```python
from build123d import *

# Parameters (mm, degrees)
SKETCH_1_W      = 134.3
SKETCH_1_H      = 22
EXTRUDE_1_DEPTH = 8
SKETCH_2_W      = 4
SKETCH_2_H      = 8
EXTRUDE_2_DEPTH = 130


with BuildPart() as part:
    # 草图1 → 凸台-拉伸1 (new body)
    with BuildSketch(Plane(origin=(0, 0, 0), x_dir=(1, 0, 0), z_dir=(0, 1, 0))):
        Rectangle(SKETCH_1_W, SKETCH_1_H)
    extrude(amount=EXTRUDE_1_DEPTH)

    # 草图2 → 凸台-拉伸2 (add)
    with BuildSketch(Plane.XY):
        with Locations((-17, 4)):
            Rectangle(SKETCH_2_W, SKETCH_2_H)
    extrude(amount=EXTRUDE_2_DEPTH)


solid = part.part
```
Design review of the part built by this model. Coordinates are the model's own, in mm. A direction names the side the tool comes from. Coordinates: 2 decimals unless noted, no trailing zeros. Write each loop counter-clockwise with the first axis right and the second up, starting at its lowest first coordinate (ties: lowest second). Pieces come first, ordered by that corner, then holes.
1) Add section B-B (x = -40). Write out the cut boundary in (y, z).
2) To check wall thickness, follow L1, parallel to X at y = 4.75, z = 101; L2, parallel to Z at x = 26.5, y = 7.75. State the ranges of each line that lie inside material, in increasing order.
3) Add section C-C (z = 82). Write out the cut boundary in (x, y), plus the area to 3 significant figures.
4) Machinability: for faces 1 (the flat face through (25, 4, 11)), 2 (the flat face through (67.15, 4, 0)), 3 (the flat face through (-19, 4, 70)), which of the approach directions +Z, -Z, +X, -X, +Y, -Y give a long, thin tool a straight path to every point of the face, cutting with its end or side? Answer none if there is none.
5) Insertion check: pin 1 (4 mm diameter, centred on y = 4.5, z = 96, fed in from -X); pin 2 (3 mm diameter, centred on x = -37.5, y = 3.5, fed in from +Z). Each pin has a flat end and moves straight along its axis. Give the tip position at first contact, or say it passes through.
6) Mouldability with a two-part tool opening along Y and no side actions: class faces 4 (the flat face through (-5, 0, 7)), 5 (the flat face through (-5, 8, 7)), 6 (the flat face through (-1, 4, -11)) as +Y half, -Y half, draft (parallel to the pull), parting line (faces both ways), or undercut.
7) Add section A-A (y = 6.75). Write out the cut boundary in (x, z), plus the area to 3 significant figures.
Check result:
1. outline: (0, -11) - (8, -11) - (8, 11) - (0, 11) - close
2. L1: x = -19 to -15
2. L2: z = -11 to 11
3. outline: (-19, 0) - (-15, 0) - (-15, 8) - (-19, 8) - close
3. area: 32.0 mm2
4. face 1: +Z, +X, +Y, -Y
4. face 2: +Z, -Z, +X, +Y, -Y
4. face 3: +Z, -X, +Y, -Y
5. pin 1: stops at x = -19
5. pin 2: stops at z = 11
6. face 4: -Y half
6. face 5: +Y half
6. face 6: draft
7. outline: (-67.15, -11) - (67.15, -11) - (67.15, 11) - (-15, 11) - (-15, 130) - (-19, 130) - (-19, 11) - (-67.15, 11) - close
7. area: 3,430 mm2
